For this review, take the finished solid that the model builds, in its own axes (mm). A direction names the side the tool comes from. Round coordinates to 2 decimals unless told otherwise and drop trailing zeros. Order: outer loops, then holes, each group sorted by start corner. A loop starts at its lowest first (then second) coordinate and runs counter-clockwise, first axis right, second up. Notation, with made-up numbers: M 43,18 L 74,18 A22 cw 74,43 Z; hole C 79.25,-17 d3. An arc over 180 degrees is marked long. Answer in a Markdown table with one row per item. Add a question column.
```python
from build123d import *

# Parameters (mm, degrees)
SKETCH1_W           = 15
SKETCH1_H           = 23.84
SKETCH1_R           = 1.75
BOSS_EXTRUDE1_DEPTH = 17.25
SKETCH2_R           = 1.75
CUT_EXTRUDE1_DEPTH  = 31.367056163
CHAMFER1_SIZE       = 2.5
CUT_EXTRUDE2_DEPTH  = 1.5
CUT_EXTRUDE3_DEPTH  = 10
FILLET2_R           = 2.5


with BuildPart() as part:
    # Sketch1 → Boss-Extrude1 (new, symmetric)
    with BuildSketch(Plane(origin=(0, 0, 0), x_dir=(0, 0, -1), z_dir=(1, 0, 0))):
        Rectangle(SKETCH1_W, SKETCH1_H)
        with Locations((2.75, 5)):
            Circle(SKETCH1_R, mode=Mode.SUBTRACT)
        with Locations((2.75, -5)):
            Circle(SKETCH1_R, mode=Mode.SUBTRACT)
    extrude(amount=BOSS_EXTRUDE1_DEPTH, both=True)

    # Sketch2 → Cut-Extrude1 (cut, through all)
    with BuildSketch(Plane(origin=(0, 11.92, 0), x_dir=(1, 0, 0), z_dir=(0, 1, 0))):
        with Locations(Location((-10, -4.25, 0), (0, 0, 270))):
            Circle(SKETCH2_R)
        with Locations(Location((10, -4.25, 0), (0, 0, 270))):
            Circle(SKETCH2_R)
    extrude(amount=-CUT_EXTRUDE1_DEPTH, mode=Mode.SUBTRACT)

    # Chamfer1
    # the kernel refuses this chamfer: 2.5 mm, written as the material it takes off along each edge
    with BuildSketch(Plane(origin=(-10, 11.92, 4.25), x_dir=(0, 0, 1), z_dir=(-1, 0, 0))) as chamfer1_piece_1:
        Polygon((1.75, -CHAMFER1_SIZE), (1.75 + CHAMFER1_SIZE, 0), (1.75, 0), align=None)
    revolve(axis=Axis((-10, 11.92, 4.25), (0, 1, 0)), mode=Mode.SUBTRACT)
    with BuildSketch(Plane(origin=(10, 11.92, 4.25), x_dir=(0, 0, 1), z_dir=(-1, 0, 0))) as chamfer1_piece_2:
        Polygon((1.75, -CHAMFER1_SIZE), (1.75 + CHAMFER1_SIZE, 0), (1.75, 0), align=None)
    revolve(axis=Axis((10, 11.92, 4.25), (0, 1, 0)), mode=Mode.SUBTRACT)

    # Sketch3 → Cut-Extrude2 (cut, symmetric)
    with BuildSketch(Plane(origin=(0, -5.08, 0), x_dir=(1, 0, 0), z_dir=(0, 1, 0))):
        Polygon((-14.618802154, -4.25), (-14.618802154, -7.5), (-5.381197846, -7.5), (-5.381197846, -4.25), (-7.690598923, -0.25), (-12.309401077, -0.25), align=None)
        Polygon((14.618802154, -4.25), (12.309401077, -0.25), (7.690598923, -0.25), (5.381197846, -4.25), (5.381197846, -7.5), (14.618802154, -7.5), align=None)
    extrude(amount=CUT_EXTRUDE2_DEPTH, both=True, mode=Mode.SUBTRACT)

    # Sketch4 → Cut-Extrude3 (cut)
    with BuildSketch(Plane.XZ.offset(3.58)):
        Polygon((-13.618802154, 6.5), (-13.618802154, 7.5), (-6.381197846, 7.5), (-6.381197846, 6.5), (-6.381197846, 4.517949192), (-8.267949192, 1.25), (-11.732050808, 1.25), (-13.618802154, 4.517949192), align=None)
        Polygon((6.381197846, 6.5), (6.381197846, 7.5), (13.618802154, 7.5), (13.618802154, 6.5), (13.618802154, 4.517949192), (11.732050808, 1.25), (8.267949192, 1.25), (6.381197846, 4.517949192), align=None)
    extrude(amount=-CUT_EXTRUDE3_DEPTH, mode=Mode.SUBTRACT)

    # Fillet2
    # the kernel refuses this fillet: 2.5 mm, written as the material it adds along each edge
    with BuildSketch(Plane(origin=(-6.381197846, 6.42, -1.732050808), x_dir=(0, -1, 0), z_dir=(0, 0, 1))) as fillet2_piece_1_section:
        with BuildLine():
            CenterArc((FILLET2_R, -FILLET2_R), FILLET2_R, 90, 90)
            Line((0, -FILLET2_R), (0, 0))
            Line((0, 0), (FILLET2_R, 0))
        make_face()
    fillet2_piece_1 = extrude(amount=9.232050808, mode=Mode.PRIVATE)
    fillet2_piece_1 = fillet2_piece_1 - Plane(origin=(-10, 5.915860335, 4.25), x_dir=(0, 0, 1), z_dir=(0, 1, 0)) * Cylinder(1.75, 29, mode=Mode.PRIVATE)
    fillet2_piece_1 = split(fillet2_piece_1, bisect_by=Plane(origin=(-7.028837061, 5.915860335, 1.25), z_dir=(0, 0, 1)), keep=Keep.TOP, mode=Mode.PRIVATE)
    add(fillet2_piece_1)
    with BuildSketch(Plane(origin=(-3.256197846, 6.42, 9.930607966), x_dir=(-0.8660254037844386, 0, 0.5000000000000002), z_dir=(-0.5000000000000002, 0, -0.8660254037844386))) as fillet2_piece_2_section:
        with BuildLine():
            CenterArc((FILLET2_R, -FILLET2_R), FILLET2_R, 90, 90)
            Line((0, -FILLET2_R), (0, 0))
            Line((0, 0), (FILLET2_R, 0))
        make_face()
    fillet2_piece_2 = extrude(amount=16.273502692, mode=Mode.PRIVATE)
    fillet2_piece_2 = split(fillet2_piece_2, bisect_by=Plane(origin=(-7.669827192, 5.902188102, 7.5), z_dir=(0, 0, -1)), keep=Keep.TOP, mode=Mode.PRIVATE)
    fillet2_piece_2 = fillet2_piece_2 - Plane(origin=(-10, 5.902188102, 4.25), x_dir=(0, 0, 1), z_dir=(0, 1, 0)) * Cylinder(1.75, 43, mode=Mode.PRIVATE)
    fillet2_piece_2 = split(fillet2_piece_2, bisect_by=Plane(origin=(-7.669827192, 5.902188102, 1.25), z_dir=(0, 0, 1)), keep=Keep.TOP, mode=Mode.PRIVATE)
    add(fillet2_piece_2)
    with BuildSketch(Plane(origin=(-2.017949192, 6.42, 1.25), x_dir=(0, 0, 1), z_dir=(-1, 0, 0))) as fillet2_piece_3_section:
        with BuildLine():
            CenterArc((FILLET2_R, -FILLET2_R), FILLET2_R, 90, 90)
            Line((0, -FILLET2_R), (0, 0))
            Line((0, 0), (FILLET2_R, 0))
        make_face()
    fillet2_piece_3 = extrude(amount=15.964101615, mode=Mode.PRIVATE)
    fillet2_piece_3 = fillet2_piece_3 - Plane(origin=(-10, 5.877722241, 4.25), x_dir=(0, 0, 1), z_dir=(0, 1, 0)) * Cylinder(1.75, 42, mode=Mode.PRIVATE)
    fillet2_piece_3 = split(fillet2_piece_3, bisect_by=Plane(origin=(-11.54711457, 5.877722241, 0.92968104), z_dir=(0.8660254037844384, 0, 0.5000000000000006)), keep=Keep.TOP, mode=Mode.PRIVATE)
    add(fillet2_piece_3)
    with BuildSketch(Plane(origin=(-8.607050808, 6.42, -4.162658774), x_dir=(0.8660254037844384, 0, 0.5000000000000004), z_dir=(-0.5000000000000006, 0, 0.8660254037844384))) as fillet2_piece_4_section:
        with BuildLine():
            CenterArc((FILLET2_R, -FILLET2_R), FILLET2_R, 90, 90)
            Line((0, -FILLET2_R), (0, 0))
            Line((0, 0), (FILLET2_R, 0))
        make_face()
    fillet2_piece_4 = extrude(amount=16.273502692, mode=Mode.PRIVATE)
    fillet2_piece_4 = split(fillet2_piece_4, bisect_by=Plane(origin=(-12.330172795, 5.902188104, 7.5), z_dir=(0, 0, -1)), keep=Keep.TOP, mode=Mode.PRIVATE)
    fillet2_piece_4 = fillet2_piece_4 - Plane(origin=(-10, 5.902188104, 4.25), x_dir=(0, 0, 1), z_dir=(0, 1, 0)) * Cylinder(1.75, 43, mode=Mode.PRIVATE)
    fillet2_piece_4 = split(fillet2_piece_4, bisect_by=Plane(origin=(-12.330172795, 5.902188104, 1.25), z_dir=(0, 0, 1)), keep=Keep.TOP, mode=Mode.PRIVATE)
    add(fillet2_piece_4)
    with BuildSketch(Plane(origin=(-13.618802154, 6.42, 7.5), x_dir=(1, 0, 0), z_dir=(0, 0, -1))) as fillet2_piece_5_section:
        with BuildLine():
            CenterArc((FILLET2_R, FILLET2_R), FILLET2_R, 180, 90)
            Line((0, FILLET2_R), (0, 0))
            Line((0, 0), (FILLET2_R, 0))
        make_face()
    fillet2_piece_5 = extrude(amount=9.232050808, mode=Mode.PRIVATE)
    fillet2_piece_5 = fillet2_piece_5 - Plane(origin=(-10, 5.915860467, 4.25), x_dir=(0, 0, 1), z_dir=(0, 1, 0)) * Cylinder(1.75, 29, mode=Mode.PRIVATE)
    fillet2_piece_5 = split(fillet2_piece_5, bisect_by=Plane(origin=(-13.860643718, 5.915860467, 4.936831069), z_dir=(0.8660254037844384, 0, 0.5000000000000006)), keep=Keep.TOP, mode=Mode.PRIVATE)
    add(fillet2_piece_5)
    with BuildSketch(Plane(origin=(13.618802154, 6.42, -1.732050808), x_dir=(0, -1, 0), z_dir=(0, 0, 1))) as fillet2_piece_6_section:
        with BuildLine():
            CenterArc((FILLET2_R, -FILLET2_R), FILLET2_R, 90, 90)
            Line((0, -FILLET2_R), (0, 0))
            Line((0, 0), (FILLET2_R, 0))
        make_face()
    fillet2_piece_6 = extrude(amount=9.232050808, mode=Mode.PRIVATE)
    fillet2_piece_6 = fillet2_piece_6 - Plane(origin=(10, 5.915860335, 4.25), x_dir=(0, 0, 1), z_dir=(0, 1, 0)) * Cylinder(1.75, 29, mode=Mode.PRIVATE)
    fillet2_piece_6 = split(fillet2_piece_6, bisect_by=Plane(origin=(12.971162939, 5.915860335, 1.25), z_dir=(0, 0, 1)), keep=Keep.TOP, mode=Mode.PRIVATE)
    add(fillet2_piece_6)
    with BuildSketch(Plane(origin=(16.743802154, 6.42, 9.930607966), x_dir=(-0.8660254037844389, 0, 0.49999999999999956), z_dir=(-0.4999999999999996, 0, -0.8660254037844389))) as fillet2_piece_7_section:
        with BuildLine():
            CenterArc((FILLET2_R, -FILLET2_R), FILLET2_R, 90, 90)
            Line((0, -FILLET2_R), (0, 0))
            Line((0, 0), (FILLET2_R, 0))
        make_face()
    fillet2_piece_7 = extrude(amount=16.273502692, mode=Mode.PRIVATE)
    fillet2_piece_7 = split(fillet2_piece_7, bisect_by=Plane(origin=(12.330172808, 5.902188102, 7.5), z_dir=(0, 0, -1)), keep=Keep.TOP, mode=Mode.PRIVATE)
    fillet2_piece_7 = fillet2_piece_7 - Plane(origin=(10, 5.902188102, 4.25), x_dir=(0, 0, 1), z_dir=(0, 1, 0)) * Cylinder(1.75, 43, mode=Mode.PRIVATE)
    fillet2_piece_7 = split(fillet2_piece_7, bisect_by=Plane(origin=(12.330172808, 5.902188102, 1.25), z_dir=(0, 0, 1)), keep=Keep.TOP, mode=Mode.PRIVATE)
    add(fillet2_piece_7)
    with BuildSketch(Plane(origin=(17.982050808, 6.42, 1.25), x_dir=(0, 0, 1), z_dir=(-1, 0, 0))) as fillet2_piece_8_section:
        with BuildLine():
            CenterArc((FILLET2_R, -FILLET2_R), FILLET2_R, 90, 90)
            Line((0, -FILLET2_R), (0, 0))
            Line((0, 0), (FILLET2_R, 0))
        make_face()
    fillet2_piece_8 = extrude(amount=15.964101615, mode=Mode.PRIVATE)
    fillet2_piece_8 = fillet2_piece_8 - Plane(origin=(10, 5.877722241, 4.25), x_dir=(0, 0, 1), z_dir=(0, 1, 0)) * Cylinder(1.75, 42, mode=Mode.PRIVATE)
    fillet2_piece_8 = split(fillet2_piece_8, bisect_by=Plane(origin=(11.547114576, 5.877722241, 0.92968105), z_dir=(-0.8660254037844389, 0, 0.4999999999999996)), keep=Keep.TOP, mode=Mode.PRIVATE)
    add(fillet2_piece_8)
    with BuildSketch(Plane(origin=(11.392949192, 6.42, -4.162658774), x_dir=(0.8660254037844389, 0, 0.49999999999999956), z_dir=(-0.4999999999999996, 0, 0.8660254037844389))) as fillet2_piece_9_section:
        with BuildLine():
            CenterArc((FILLET2_R, -FILLET2_R), FILLET2_R, 90, 90)
            Line((0, -FILLET2_R), (0, 0))
            Line((0, 0), (FILLET2_R, 0))
        make_face()
    fillet2_piece_9 = extrude(amount=16.273502692, mode=Mode.PRIVATE)
    fillet2_piece_9 = split(fillet2_piece_9, bisect_by=Plane(origin=(7.669827205, 5.902188104, 7.5), z_dir=(0, 0, -1)), keep=Keep.TOP, mode=Mode.PRIVATE)
    fillet2_piece_9 = fillet2_piece_9 - Plane(origin=(10, 5.902188104, 4.25), x_dir=(0, 0, 1), z_dir=(0, 1, 0)) * Cylinder(1.75, 43, mode=Mode.PRIVATE)
    fillet2_piece_9 = split(fillet2_piece_9, bisect_by=Plane(origin=(7.669827205, 5.902188104, 1.25), z_dir=(0, 0, 1)), keep=Keep.TOP, mode=Mode.PRIVATE)
    add(fillet2_piece_9)
    with BuildSketch(Plane(origin=(6.381197846, 6.42, 7.5), x_dir=(1, 0, 0), z_dir=(0, 0, -1))) as fillet2_piece_10_section:
        with BuildLine():
            CenterArc((FILLET2_R, FILLET2_R), FILLET2_R, 180, 90)
            Line((0, FILLET2_R), (0, 0))
            Line((0, 0), (FILLET2_R, 0))
        make_face()
    fillet2_piece_10 = extrude(amount=9.232050808, mode=Mode.PRIVATE)
    fillet2_piece_10 = fillet2_piece_10 - Plane(origin=(10, 5.915860467, 4.25), x_dir=(0, 0, 1), z_dir=(0, 1, 0)) * Cylinder(1.75, 29, mode=Mode.PRIVATE)
    fillet2_piece_10 = split(fillet2_piece_10, bisect_by=Plane(origin=(6.139356282, 5.915860467, 4.936831069), z_dir=(0.8660254037844389, 0, 0.4999999999999996)), keep=Keep.TOP, mode=Mode.PRIVATE)
    add(fillet2_piece_10)


solid = part.part
```
1. Consider section C-C on y = -5. Write out the cut boundary in (x, z), plus the area to 3 significant figures.
2. Consider section D-D on y = 1. Write out the cut boundary in (x, z), plus the area to 3 significant figures.
3. For faces 1 (the flat face through (5.381, -5, 6)), 2 (the cylindrical face through (-0.24, -6.55, -3.56)), list the 3-axis set-ups (+Z, -Z, +X, -X, +Y, -Y) from which the entire face can be reached by the end or side of a thin tool; tool diameter is ignored.
4. Consider section B-B on x = 5. Write out the cut boundary in (y, z).
5. The part is to be moulded in two halves that separate along X. For faces 3 (the flat face through (10, 6.42, 7)), 4 (the flat face through (0, 0, 7.5)), 5 (the flat face through (17.25, 0, 0)), say which applies: pulls with the +X half, pulls with the -X half, needs draft (parallel to the pull), parting line crosses it, or undercut.
6. Consider section A-A on z = -2.75. Write out the cut boundary in (x, y), plus the area to 3 significant figures.
7. Clearance check with flat-ended pins moving along their axes: pin 1 Ø4 at (x, z) = (-10, 4.25) entering from +Y; pin 2 Ø3.5 at (x, z) = (9, 4.5) entering from +Y; pin 3 Ø3 at (x, y) = (9.5, -0.5) entering from +Z; pin 4 Ø3 at (y, z) = (-5, -2.75) entering from +X. State where each tip first meets the part, or that it passes through.
8. To check wall thickness, follow probe 1 along X at (y, z) = (-1.5, 5.75); probe 2 along X at (y, z) = (-8.75, 4.25); probe 3 along Y at (x, z) = (-4, -2.75). State the ranges of each line that lie inside material, in increasing order. Write a range as [from, to].
Solved:
| question | item | result |
|---|---|---|
| 1 | outline | M -17.25,-7.5 L 17.25,-7.5 L 17.25,-4.5 L -17.25,-4.5 Z; M -17.25,-1 L 17.25,-1 L 17.25,7.5 L 14.62,7.5 L 14.62,4.25 L 12.31,0.25 L 7.69,0.25 L 5.38,4.25 L 5.38,7.5 L -5.38,7.5 L -5.38,4.25 L -7.69,0.25 L -12.31,0.25 L -14.62,4.25 L -14.62,7.5 L -17.25,7.5 Z |
| 1 | area | 281 mm^2 |
| 2 | outline | M -17.25,-7.5 L 17.25,-7.5 L 17.25,7.5 L 13.62,7.5 L 13.62,4.52 L 11.73,1.25 L 8.27,1.25 L 6.38,4.52 L 6.38,7.5 L -6.38,7.5 L -6.38,4.52 L -8.27,1.25 L -11.73,1.25 L -13.62,4.52 L -13.62,7.5 L -17.25,7.5 Z |
| 2 | area | 439 mm^2 |
| 3 | face 1 | +Z |
| 3 | face 2 | +X, -X |
| 4 | outline | M -11.92,-7.5 L 11.92,-7.5 L 11.92,7.5 L -11.92,7.5 Z; hole C -5,-2.75 d3.5; hole C 5,-2.75 d3.5 |
| 5 | face 3 | undercut |
| 5 | face 4 | needs draft |
| 5 | face 5 | pulls with the +X half |
| 6 | outline | M -17.25,-11.92 L 17.25,-11.92 L 17.25,-6.75 L -17.25,-6.75 Z; M -17.25,-3.25 L 17.25,-3.25 L 17.25,3.25 L -17.25,3.25 Z; M -17.25,6.75 L 17.25,6.75 L 17.25,11.92 L -17.25,11.92 Z |
| 6 | area | 581 mm^2 |
| 7 | pin 1 | stops at y = 9.67 |
| 7 | pin 2 | stops at y = 10.45 |
| 7 | pin 3 | stops at z = 1.71 |
| 7 | pin 4 | passes through |
| 8 | probe 1 | x = [-17.25, -13.62], [-6.38, 6.38], [13.62, 17.25] |
| 8 | probe 2 | x = [-17.25, -11.75], [-8.25, 8.25], [11.75, 17.25] |
| 8 | probe 3 | y = [-11.92, -6.75], [-3.25, 3.25], [6.75, 11.92] |
